Can you work these out from the model? Positions are in its coordinate system, mm. A direction names the side the tool comes from. Give positions to 0.01 mm unless a question says otherwise; leave off trailing zeros. Write each loop counter-clockwise with the first axis right and the second up, starting at its lowest first coordinate (ties: lowest second). Pieces come first, ordered by that corner, then holes. Notation, with made-up numbers: (72, -20.75) -> (110, -20.75) arc R24 ccw to (110, -4.75) -> close; hole circle Ø3 at (54.5, -15). An arc over 180 degrees is marked (long way). One line per item, written item: value.
from build123d import *

# Parameters (mm, degrees)
F0_W     = 50
F0_H     = 50
F1_DEPTH = 10
F2_W     = 30
F2_H     = 8
F3_DEPTH = 40
F4_W     = 30
F4_H     = 8
F5_DEPTH = 30
F7_DEPTH = 8
F9_R     = 14.99999
F11_D    = 5


# Not quite as in the source:
# - a fillet or chamfer is up to 0.001 mm smaller than in the source, because OpenCascade refuses the exact size


with BuildPart() as f1:
    # F0 (on Top) → F1 (new body)
    with BuildSketch(Plane.XY):
        with Locations((1.1680293828, -3.1129003775)):
            Rectangle(F0_W, F0_H)
    extrude(amount=F1_DEPTH)

    # F2 (on face) → F3 (join)
    with BuildSketch(Plane.XY.offset(10)):
        with Locations((1.5573729761, 7.8870996225)):
            Rectangle(F2_W, F2_H)
    extrude(amount=F3_DEPTH)

    # F4 (on face) → F5 (join)
    with BuildSketch(Plane.XY.offset(10)):
        with Locations((1.5573729761, -14.1129003775)):
            Rectangle(F4_W, F4_H)
    extrude(amount=F5_DEPTH)

    # F6 (on face) → F7 (join)
    with BuildSketch(Plane.XZ.offset(18.1129003775)):
        with BuildLine():
            Line((-13.4426270239, 40), (16.5573729761, 40))
            ThreePointArc((16.5573729761, 40), (1.5573729761, 49.8339152222), (-13.4426270239, 40))
        make_face()
    extrude(amount=-F7_DEPTH)

    # F9 (radius 15 in the source; OpenCascade refuses exactly that, so slightly less here)
    f9_edges = [f1.edges().sort_by_distance(p)[0] for p in [
        (16.557373, 7.8871, 50),
        (-13.442627, 7.8871, 50),
    ]]
    fillet(f9_edges, radius=F9_R)

    # F11 (through all)
    with Locations(Plane.XZ.offset(18.1129003775)):
        with Locations((1.6286504688, 40.3330288827)):
            Hole(F11_D / 2)


solid = f1.part
1) If we section it at B-B (x = -8.5): Write out the boundary of the cut face in (y, z), and give its area (3 significant figures).
Answer list:
outline: (-28.11, 0) -> (21.89, 0) -> (21.89, 10) -> (11.89, 10) -> (11.89, 46.13) -> (3.89, 46.13) -> (3.89, 10) -> (-10.11, 10) -> (-10.11, 46.38) -> (-18.11, 46.38) -> (-18.11, 10) -> (-28.11, 10) -> close
area: 1,080 mm^2
2) If we section it at A-A (z = 12.5): Write out the boundary of the cut face in (x, y).
Answer list:
outline: (-13.44, -18.11) -> (16.56, -18.11) -> (16.56, -10.11) -> (-13.44, -10.11) -> close; (-13.44, 3.89) -> (16.56, 3.89) -> (16.56, 11.89) -> (-13.44, 11.89) -> close
3) If we section it at D-D (z = 44): Write out the boundary of the cut face in (x, y), and give its area (3 significant figures).
Answer list:
outline: (-10.97, -18.11) -> (14.08, -18.11) -> (14.08, -10.11) -> (-10.97, -10.11) -> close; (-10.44, 3.89) -> (13.56, 3.89) -> (13.56, 11.89) -> (-10.44, 11.89) -> close
area: 392 mm^2
4) Will these pins go through, and if not, where does the flat tip stop? pin 1 (10 mm diameter, centred on x = 9.5, z = 24, fed in from -Y); pin 2 (25 mm diameter, centred on x = 9, y = 8, fed in from +Z); pin 3 (2.5 mm diameter, centred on y = 6.5, z = 23, fed in from -X); pin 4 (15 mm diameter, centred on x = -5, z = 35.5, fed in from +Y).
Answer list:
pin 1: stops at y = -18.11
pin 2: stops at z = 50
pin 3: stops at x = -13.44
pin 4: stops at y = 11.89
5) I need wall thicknesses on L1, parallel to Y at x = 6.5, z = 12.5; L2, parallel to Z at x = 14.5, y = -21; L3, parallel to X at y = -15, z = 28. Which ranges of each line are inside material? Lowest first, please.
Answer list:
L1: y = -18.11 to -10.11, 3.89 to 11.89
L2: z = 0 to 10
L3: x = -13.44 to 16.56
6) If we section it at C-C (y = -4.5): Write out the boundary of the cut face in (x, z), and give its area (3 significant figures).
Answer list:
outline: (-23.83, 0) -> (26.17, 0) -> (26.17, 10) -> (-23.83, 10) -> close
area: 500 mm^2
7) For faces 5 (the face through (1, -18.113, 30)), 6 (the face through (1.82, -14.17, 49.83)), 7 (the face through (-13.443, 8, 22)), 8 (the face through (16.557, 8, 22)), which set-ups out of +Z, -Z, +X, -X, +Y, -Y let a thin tool reach every point of the face, with its end or its side?
Answer list:
face 5: +Z, +X, -X, -Y
face 6: +Z, -Y
face 7: +Z, -X, +Y, -Y
face 8: +Z, +X, +Y, -Y
8) We'd pull the mould along Y, two halves only. Please class faces 1 (the face through (1, -10.113, 30)), 2 (the face through (1, 21.887, 5)), 3 (the face through (1, 3.887, 30)), 4 (the face through (16.557, -14, 25)): released by +Y, released by -Y, zero draft, split by the parting line, or undercut.
Answer list:
face 1: undercut
face 2: released by +Y
face 3: undercut
face 4: zero draft
